```python
from build123d import *

# Parameters (mm, degrees)
EXTRUDE3_DEPTH     = 1.524
SKETCH4_W          = 25.4
SKETCH4_H          = 1.4224
CHAMFER2_SIZE      = 0.47625
SKETCH26_R         = 0.5461
EXTRUDE12_DEPTH    = 1.524
SKETCH30_OUTSIDE_W = 21.138
SKETCH30_OUTSIDE_H = 21.876
SKETCH30_OUTSIDE_R = 2.38125
EXTRUDE13_DEPTH    = 2.54
EXTRUDE13_DRAFT    = -60


with BuildPart() as part:
    # Sketch1 → Extrude3 (new body)
    with BuildSketch(Plane.XY):
        Polygon((-2.38125, -1.374815329), (0, -2.749630657), (2.38125, -1.374815329), (2.38125, 1.374815329), (0, 2.749630657), (-2.38125, 1.374815329), align=None)
    extrude(amount=EXTRUDE3_DEPTH)



with BuildPart() as body_2:
    # Sketch4 → Revolve1 (revolve)
    with BuildSketch(Plane(origin=(0, 0, 0), x_dir=(0, 0, -1), z_dir=(1, 0, 0)), mode=Mode.PRIVATE) as revolve1_sk:
        with Locations((12.7, 0.7112)):
            Rectangle(SKETCH4_W, SKETCH4_H)
    revolve(revolve1_sk.sketch.rotate(Axis((0, 0, 0), (0, 0, -1)), 90), axis=Axis((0, 0, 0), (0, 0, -1)))

    # Chamfer2
    chamfer2_edges = [body_2.edges().sort_by_distance(p)[0] for p in [
        (-1.4224, 0, -25.4),
    ]]
    chamfer(chamfer2_edges, length=CHAMFER2_SIZE)


with BuildPart() as part_1:
    add(part.part)

    add(body_2.part)  # Extrude12 merges body 2
    # Sketch26 → Extrude12 (add)
    with BuildSketch(Plane.XY):
        Circle(SKETCH26_R)
    extrude(amount=EXTRUDE12_DEPTH)


with BuildPart() as extrude13_tool:
    # Sketch30 outside → Extrude13 (with draft: the straight prism first)
    with BuildSketch(Plane.XY.offset(1.524)):
        Rectangle(SKETCH30_OUTSIDE_W, SKETCH30_OUTSIDE_H)
        Circle(SKETCH30_OUTSIDE_R, mode=Mode.SUBTRACT)
    extrude(amount=-EXTRUDE13_DEPTH)
    # Extrude13: the draft: its side faces are tilted about the plane it starts from
    extrude13_sides = [extrude13_tool.faces().sort_by_distance(p)[0] for p in [
        (0, -10.938, 0.254),
        (10.569, 0, 0.254),
        (0, 10.938, 0.254),
        (-10.569, 0, 0.254),
        (-2.38125, 0, 0.254),
    ]]
    draft(extrude13_sides, Plane.XY.offset(1.524), EXTRUDE13_DRAFT)


with BuildPart() as part_2:
    add(part_1.part)

    # Extrude13: cut by extrude13_tool
    add(extrude13_tool.part, mode=Mode.SUBTRACT)


solid = part_2.part
```
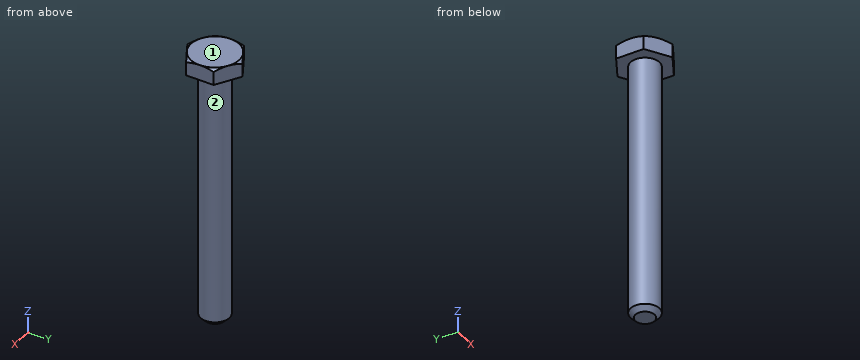
Input: part model. Units: mm. Frame: model coordinates. Face numbers are marked on the shaded views. A direction names the side the tool comes from. Coordinates: 2 decimals unless noted, no trailing zeros. Order: outer loops, then holes, each group sorted by start corner. A loop starts at its lowest first (then second) coordinate and runs counter-clockwise, first axis right, second up. Notation, with made-up numbers: (71, 18.25) - (83, 18.25) arc R30 cw to (83, 42.25) - close; hole circle Ø7 at (-25, -36). An arc over 180 degrees is marked (long way). Return JSON: item names as keys, results as strings.
Q1. Access query for the marked faces 1 and 2. Directions: +Z, -Z, +X, -X, +Y, -Y. A direction counts if a zero-diameter tool reaches every point of the face in a straight line with its end or side. Return the directions, or none.
The answers:
{"face 1": "+Z, +X, -X, +Y, -Y", "face 2": "-Z"}
Q2. First-contact query: pin 1 (2 mm diameter, centred on x = -1.5, y = -1.5, fed in from -Z); pin 2 (1 mm diameter, centred on x = 1.5, y = -0.5, fed in from -Z) (3 decimals). Flat tips, straight axial feed; report the tip coordinate or a pass-through.
The answers:
{"pin 1": "stops at z = -25.22", "pin 2": "stops at z = -25.265"}
Q3. Cut plane A-A (z = -18.25). Return loops of the section in (x, y).
The answers:
{"outline": "circle Ø2.84 at (0, 0)"}
Q4. Ray query, probe 1 along Z at (x, y) = (0.9, 1.6); probe 2 along X at (y, z) = (-0.35, -7.25); probe 3 along Y at (x, z) = (-0.8, -8.5). Return the intervals inside material, ascending.
The answers:
{"probe 1": "z = 0 to 1.52", "probe 2": "x = -1.38 to 1.38", "probe 3": "y = -1.18 to 1.18"}
